Work out the finished part from the listing and answer in its coordinate system (mm). A direction names the side the tool comes from. Round coordinates to 2 decimals unless told otherwise and drop trailing zeros. Order: outer loops, then holes, each group sorted by start corner. A loop starts at its lowest first (then second) coordinate and runs counter-clockwise, first axis right, second up. Notation, with made-up numbers: (89.25, 76) - (128.25, 76) arc R12 cw to (128.25, 82) - close; hole circle Ø11 at (55.25, 58). An arc over 180 degrees is marked (long way). Put each result on its own line as item: value.
Autodesk Inventor part; units mm, degrees
ref_plane "YZ Plane" through (0, 0, 0) normal (1, 0, 0) x (0, 1, 0)
ref_plane "XZ Plane" through (0, 0, 0) normal (0, 1, 0) x (-1, 0, 0)
ref_plane "XY Plane" through (0, 0, 0) normal (0, 0, 1) x (1, 0, 0)
sketch "Sketch1" plane through (0, 0, 0) normal (0, 0, 1) x (1, 0, 0)
  line L0 (2.7424, 0) -> (1.3712, -2.375)
  line L1 (1.3712, -2.375) -> (-1.3712, -2.375)
  line L2 (-1.3712, -2.375) -> (-2.7424, 0)
  line L3 (-2.7424, 0) -> (-1.3712, 2.375)
  line L4 (-1.3712, 2.375) -> (1.3712, 2.375)
  line L5 (1.3712, 2.375) -> (2.7424, 0)
  point P0 (0, 0)
  point P1 (0, 0)
  dimension "d0" = 4.75
extrude "Extrusion1" add sketch "Sketch1" along normal blind 4.8
sketch "Sketch2" plane through (0, 0, 0) normal (0, 0, -1) x (-1, 0, 0)
  circle A0 centre (0, 0) radius 1.4
  dimension "d3" = 2.8
extrude "Extrusion2" add sketch "Sketch2" along normal blind 6
sketch "Sketch3" plane through (0, 0, 4.8) normal (0, 0, 1) x (1, 0, 0)
  circle A0 centre (0, 0) radius 1.2
  dimension "d6" = 2.4
extrude "Extrusion3" cut sketch "Sketch3" against normal blind 4
fillet "Fillet1" radius 0.5 6 edges at (-2.7424, 0, 2.4) (-1.3712, -2.375, 2.4) (1.3712, -2.375, 2.4) (2.7424, 0, 2.4) (1.3712, 2.375, 2.4) (-1.3712, 2.375, 2.4)
fillet "Fillet2" radius 0.2 12 edges at (-2.0568, 1.1875, 4.8) (-2.6651, 0, 4.8) (-2.0568, -1.1875, 4.8) (-1.3325, -2.308, 4.8) (0, -2.375, 4.8) (1.3325, -2.308, 4.8) (2.0568, -1.1875, 4.8) (2.6651, 0, 4.8) (2.0568, 1.1875, 4.8) (1.3325, 2.308, 4.8) (0, 2.375, 4.8) (-1.3325, 2.308, 4.8)
properties part number "5207953-3"
1) For a pull along Y with two mould halves and no side action, classify faces 4 (the cylindrical face through (0.65, 1.01, 2.83)), 5 (the cylindrical face through (-2.01, -1.15, 4.74)), 6 (the flat face through (0, 0, -6)), 7 (the cylindrical face through (1.4, -0.06, -2.96)) as pulls with the +Y half, pulls with the -Y half, needs draft (parallel to the pull), parting line crosses it, or undercut.
Findings below:
face 4: undercut
face 5: pulls with the -Y half
face 6: needs draft
face 7: parting line crosses it
2) A cutting plane is placed at D-D on z = -1. Write down the section's boundary in (x, y).
Findings below:
outline: circle Ø2.8 at (0, 0)
3) A cutting plane is placed at C-C on x = 0. Write down the section's boundary in (y, z) (3 decimals).
Findings below:
outline: (-2.375, 0) - (-1.4, 0) - (-1.4, -6) - (1.4, -6) - (1.4, 0) - (2.375, 0) - (2.375, 4.6) arc R0.2 ccw to (2.175, 4.8) - (1.2, 4.8) - (1.2, 0.8) - (-1.2, 0.8) - (-1.2, 4.8) - (-2.175, 4.8) arc R0.2 ccw to (-2.375, 4.6) - close
4) For faces 1 (the flat face through (2.05, 1.2, 2.27)), 2 (the flat face through (0, -2, 0)), 3 (the flat face through (0, 0, 0.8)), determine the directions among +Z, -Z, +X, -X, +Y, -Y from which every point of the face is accessible in a straight line to the end or side of a thin tool.
Findings below:
face 1: +Z, -Z, +X, +Y
face 2: -Z
face 3: +Z
5) Straight lines are drawn through the part: L1, parallel to Y at x = 0, z = 2.2 (3 decimals); L2, parallel to Z at x = -0.55, y = 2.1; L3, parallel to X at y = -0.8, z = 3. For each, find the intervals that lie inside material, in ascending order. Write a range as from..to.
Findings below:
L1: y = -2.375..-1.2, 1.2..2.375
L2: z = 0..4.8
L3: x = -2.28..-0.89, 0.89..2.28
6) A cutting plane is placed at B-B on y = 0. Write down the section's boundary in (x, z), then the cut area to 3 significant figures.
Findings below:
outline: (-2.67, 0) - (-1.4, 0) - (-1.4, -6) - (1.4, -6) - (1.4, 0) - (2.67, 0) - (2.67, 4.6) arc R0.2 ccw to (2.47, 4.8) - (1.2, 4.8) - (1.2, 0.8) - (-1.2, 0.8) - (-1.2, 4.8) - (-2.47, 4.8) arc R0.2 ccw to (-2.67, 4.6) - close
area: 32.8 mm2
7) A cutting plane is placed at A-A on z = 1.25. Write down the section's boundary in (x, y) (3 decimals).
Findings below:
outline: (-2.598, -0.25) - (-1.516, -2.125) arc R0.5 ccw to (-1.083, -2.375) - (1.083, -2.375) arc R0.5 ccw to (1.516, -2.125) - (2.598, -0.25) arc R0.5 ccw to (2.598, 0.25) - (1.516, 2.125) arc R0.5 ccw to (1.083, 2.375) - (-1.083, 2.375) arc R0.5 ccw to (-1.516, 2.125) - (-2.598, 0.25) arc R0.5 ccw to start; hole circle Ø2.4 at (0, 0)
